from build123d import *

# Parameters (mm, degrees)
SKETCH1_R           = 12.7
BOSS_EXTRUDE1_DEPTH = 50
SKETCH2_R           = 6.35
CUT_EXTRUDE1_DEPTH  = 51
FILLET1_R           = 5


with BuildPart() as part:
    # Sketch1 → Boss-Extrude1 (new body)
    with BuildSketch(Plane(origin=(0, 0, 0), x_dir=(0, 0, -1), z_dir=(1, 0, 0))):
        Circle(SKETCH1_R)
    extrude(amount=BOSS_EXTRUDE1_DEPTH)

    # Sketch2 → Cut-Extrude1 (cut, through all)
    with BuildSketch(Plane(origin=(50, 0, 0), x_dir=(0, 0, -1), z_dir=(1, 0, 0))):
        Circle(SKETCH2_R)
    extrude(amount=-CUT_EXTRUDE1_DEPTH, mode=Mode.SUBTRACT)

    # Fillet1
    fillet1_edges = [part.edges().sort_by_distance(p)[0] for p in [
        (50, 0, 6.35),
    ]]
    fillet(fillet1_edges, radius=FILLET1_R)


solid = part.part
Geometry check sheet. Reference: the model listing, model coordinates, mm. Coordinates: 2 decimals unless noted, no trailing zeros. Order: outer loops, then holes, each group sorted by start corner. A loop starts at its lowest first (then second) coordinate and runs counter-clockwise, first axis right, second up. Notation, with made-up numbers: (83.5, 58) - (107.5, 58) arc R28 cw to (107.5, 81) - close; hole circle Ø3 at (55, 45.5). An arc over 180 degrees is marked (long way). One line per item, written item: value.
(1) Release check for a two-part mould opening along Z. For faces 1 (the face through (24.65, -12.4, 2.75)), 2 (the face through (22.82, -6.2, 1.38)), 3 (the face through (0, 6, -3)) record: +Z half, -Z half, draft (parallel to the pull), parting line (faces both ways), or undercut.
Data:
face 1: parting line
face 2: undercut
face 3: draft
(2) Sectioned sample at C-C (x = 42). Enter the section's corners in (y, z).
Data:
outline: circle Ø25.4 at (0, 0); hole circle Ø12.7 at (0, 0)
(3) Depth check by flat-ended pin: pin 1 Ø1.5 at (x, y) = (7.5, -8.5) entering from +Z; pin 2 Ø12 at (x, z) = (14, 6) entering from -Y; pin 3 Ø1.5 at (x, z) = (31, 9) entering from -Y; pin 4 Ø5 at (y, z) = (2, -0.5) entering from +X. Enter the tip coordinate at first touch or a pass-through.
Data:
pin 1: stops at z = 10.06
pin 2: stops at y = -12.7
pin 3: stops at y = -9.66
pin 4: passes through
(4) Sectioned sample at A-A (y = 0). Enter the section's corners in (x, z).
Data:
outline: (0, -12.7) - (50, -12.7) - (50, -11.35) arc R5 ccw to (45, -6.35) - (0, -6.35) - close; (0, 6.35) - (45, 6.35) arc R5 ccw to (50, 11.35) - (50, 12.7) - (0, 12.7) - close
(5) Thickness scan on probe 1 along Y at (x, z) = (30.5, 0); probe 2 along Z at (x, y) = (46, 5.75); probe 3 along Y at (x, z) = (44, 3). Record the ranges inside material, lowest first. Write a range as from..to.
Data:
probe 1: y = -12.7..-6.35, 6.35..12.7
probe 2: z = -11.32..-2.92, 2.92..11.32
probe 3: y = -12.34..-5.6, 5.6..12.34
